```python
from build123d import *

# Parameters (mm, degrees)
SKETCH1_W           = 25.4
SKETCH1_H           = 12.7
BOSS_EXTRUDE1_DEPTH = 460.375
SKETCH2_W           = 6.35
SKETCH2_H           = 25.4
CUT_EXTRUDE1_DEPTH  = 462.250030488
SKETCH3_R           = 6.35
CUT_EXTRUDE2_DEPTH  = 462.11888177


with BuildPart() as part:
    # Sketch1 → Boss-Extrude1 (new body)
    with BuildSketch(Plane(origin=(0, 0, 0), x_dir=(1, 0, 0), z_dir=(0, 1, 0))):
        with Locations((12.7, 6.35)):
            Rectangle(SKETCH1_W, SKETCH1_H)
    extrude(amount=BOSS_EXTRUDE1_DEPTH)

    # Sketch2 → Cut-Extrude1 (cut, through all)
    with BuildSketch(Plane(origin=(25.4, 0, 0), x_dir=(0, 0, -1), z_dir=(1, 0, 0))):
        with Locations((3.175, 441.325)):
            Rectangle(SKETCH2_W, SKETCH2_H)
        with Locations((3.175, 19.05)):
            Rectangle(SKETCH2_W, SKETCH2_H)
    extrude(amount=-CUT_EXTRUDE1_DEPTH, mode=Mode.SUBTRACT)

    # Sketch3 → Cut-Extrude2 (cut, through all)
    with BuildSketch(Plane.XY.offset(-6.35)):
        with Locations((12.7, 441.325)):
            Circle(SKETCH3_R)
        with Locations((12.7, 19.05)):
            Circle(SKETCH3_R)
    extrude(amount=-CUT_EXTRUDE2_DEPTH, mode=Mode.SUBTRACT)


solid = part.part
```
Geometry: final body of the model. Coordinates: model frame, mm. A direction names the side the tool comes from. Coordinates: 2 decimals unless noted, no trailing zeros. Write each loop counter-clockwise with the first axis right and the second up, starting at its lowest first coordinate (ties: lowest second). Pieces come first, ordered by that corner, then holes. Notation, with made-up numbers: M 47,50.5 L 80,50.5 A23 ccw 80,73.5 Z; hole C -29.5,-14.5 d5. An arc over 180 degrees is marked long. Answer as CSV lines item,"result". Start each with the question number.
Q1. Cut plane C-C on x = 12.7. Return the cut outline in (y, z) (3 decimals), then the cut area to 3 significant figures.
Q2. Cut plane B-B on z = -3.75. Return the cut outline in (x, y) (3 decimals), then the cut area to 3 significant figures.
Q3. Line query: line 1 (Y direction, x = 3.5, z = -4) (3 decimals); line 2 (Y direction, x = 12.7, z = -10.25) (3 decimals); line 3 (Z direction, x = 23, y = 434). Output: solid intervals per line, ascending. Write a range as from..to.
Q4. Reachability of faces 5 (the flat face through (13, 227, 0)), 6 (the flat face through (15.7, 435.5, -6.35)) from +Z, -Z, +X, -X, +Y, -Y: full face, straight path, thin tool, end or side. Return the list, or none.
Q5. Mould query, pull axis Y, two halves, no side actions, for faces 1 (the cylindrical face through (8.02, 23.34, -9.48)), 2 (the flat face through (16, 13, -6.35)), 3 (the flat face through (13, 227, -12.7)), 4 (the flat face through (13, 460.375, -6)). Classes: released by +Y, released by -Y, zero draft, split by the parting line, or undercut.
Q6. Cut plane A-A on y = 19.05. Return the cut outline in (x, z), then the cut area to 3 significant figures.
Q7. Pin query (flat end, axial travel): P1, Ø7.5, axis at x = 6.5, y = 435, coming from the +Z side; P2, Ø11.5, axis at x = 12.7, y = 19.05, coming from the +Z side. Return the tip coordinate at first contact, or that it passes through.
Findings below:
1,outline,"M 0,-12.7 L 12.7,-12.7 L 12.7,-6.35 L 6.35,-6.35 L 6.35,0 L 0,0 Z; M 25.4,-12.7 L 434.975,-12.7 L 434.975,-6.35 L 428.625,-6.35 L 428.625,0 L 31.75,0 L 31.75,-6.35 L 25.4,-6.35 Z; M 447.675,-12.7 L 460.375,-12.7 L 460.375,0 L 454.025,0 L 454.025,-6.35 L 447.675,-6.35 Z"
1,area,"5,360 mm2"
2,outline,"M 0,0 L 25.4,0 L 25.4,6.35 L 0,6.35 Z; M 0,31.75 L 25.4,31.75 L 25.4,428.625 L 0,428.625 Z; M 0,454.025 L 25.4,454.025 L 25.4,460.375 L 0,460.375 Z"
2,area,"10,400 mm2"
3,line 1,"y = 0..6.35, 31.75..428.625, 454.025..460.375"
3,line 2,"y = 0..12.7, 25.4..434.975, 447.675..460.375"
3,line 3,"z = -12.7..-6.35"
4,face 5,"+Z, +X, -X, +Y, -Y"
4,face 6,"+Z, +X, -X"
5,face 1,"undercut"
5,face 2,"undercut"
5,face 3,"zero draft"
5,face 4,"released by +Y"
6,outline,"M 0,-12.7 L 6.35,-12.7 L 6.35,-6.35 L 0,-6.35 Z; M 19.05,-12.7 L 25.4,-12.7 L 25.4,-6.35 L 19.05,-6.35 Z"
6,area,"80.6 mm2"
7,P1,"stops at z = -6.35"
7,P2,"passes through"
